from build123d import *

# Parameters (mm, degrees)
POCKET_DEPTH       = 34.402163
POCKET_DEPTH_BACK  = 40.002163
POLARPATTERN_COUNT = 6


with BuildPart() as part:
    # Sketch → Revolution (revolve)
    with BuildSketch(Plane.XZ):
        Polygon((-3.6, 4.6), (-3.6, 3.5), (-3.38, 3), (-3.6, 2.5), (-3.6, 1), (-3.405, 0.5), (-3.905, 0), (-4.4, 0), (-5.4, 0), (-5.75, 0.35), (-5.75, 1), (-4.675, 1), (-4.675, 2.3), (-4.4, 2.575), (-4.4, 4.85), (-3.65, 5.6), (-3.15, 5.6), (-2.975, 5.1), (-3.15, 4.6), align=None)
    revolve(axis=Axis((0, 0, 0), (0, 0, 1)))

    # Sketch001 → Pocket (cut, two sides)
    with BuildSketch(Plane.XY) as pocket_sk:
        with BuildLine():
            Line((0, 0), (-0.776457, 2.897777))
            ThreePointArc((-0.587735, 3.196415), (-0.747472, 3.08841), (-0.776457, 2.897777))
            ThreePointArc((0.587735, 3.196415), (0, 3.25), (-0.587735, 3.196415))
            ThreePointArc((0.776457, 2.897777), (0.747472, 3.08841), (0.587735, 3.196415))
            Line((0.776457, 2.897777), (0, 0))
        make_face()
    pocket = extrude(amount=-POCKET_DEPTH, mode=Mode.SUBTRACT) + extrude(pocket_sk.sketch, amount=POCKET_DEPTH_BACK, mode=Mode.SUBTRACT)

    # PolarPattern: Pocket ×6 about axis
    polarpattern_axis = Axis((0, 0, 0), (0, 0, 1))
    for i in range(1, POLARPATTERN_COUNT):
        add(pocket.rotate(polarpattern_axis, i * 360 / POLARPATTERN_COUNT), mode=Mode.SUBTRACT)


solid = part.part
Input: part model. Units: mm. Frame: model coordinates. A direction names the side the tool comes from. Coordinates: 2 decimals unless noted, no trailing zeros. Loops run counter-clockwise (first coordinate to the right, second up) from the corner with the lowest first, then second, coordinate; pieces in that order, holes last.
Q1. Cut plane B-B (z = 4.45). Output: boundary loops of the cut face in (x, y), then the cut area to 3 significant figures.
Q2. Contact query for flat-ended pins moving along their axis: pin 1 (2 mm diameter, centred on x = 1, y = -1.5, fed in from -Z); pin 2 (1 mm diameter, centred on y = -4.5, z = 3, fed in from +X); pin 3 (1.5 mm diameter, centred on x = 0.5, z = 5, fed in from -Y); pin 4 (1 mm diameter, centred on x = 1.5, y = -4.5, fed in from +Z). Output: stop coordinate, or through.
Q3. Draft query along Z for faces 1 (the face through (1.013, 4.564, 1.659)), 2 (the face through (-3.434, -1.081, 1.74)), 3 (the face through (-3.434, -1.081, 4.042)), 4 (the face through (-1.542, -2.647, 4.846)). Return one class per face: +Z half, -Z half, draft (parallel to the pull), parting line (faces both ways), or undercut.
Q4. Set-up query: faces 5 (the face through (-4.197, -1.322, 3.728)), 6 (the face through (0.01, 3.25, 5.09)), 7 (the face through (1.542, 2.647, 4.846)). Return all of +Z, -Z, +X, -X, +Y, -Y with unobstructed straight access to the full face (end or side cutting, diameter ignored); none if empty.
Q5. Cut plane C-C (z = 3.15). Output: boundary loops of the cut face in (x, y).
Q6. Material intervals for line 1 (X direction, y = 0, z = 3.95); line 2 (X direction, y = 0, z = 2.05) (3 decimals); line 3 (Z direction, x = 1.25, y = -3.25), sorted ascending.
Working result:
1. outline: circle Ø8.8 at (0, 0); hole circle Ø7.2 at (0, 0)
1. area: 20.1 mm2
2. pin 1: passes through
2. pin 2: stops at x = 1.83
2. pin 3: stops at y = -4.4
2. pin 4: stops at z = 5.01
3. face 1: draft
3. face 2: undercut
3. face 3: undercut
3. face 4: -Z half
4. face 5: +Z
4. face 6: +Z, -Z
4. face 7: -Z
5. outline: circle Ø8.8 at (0, 0); hole circle Ø6.89 at (0, 0)
6. line 1: x = -4.4 to -3.6, 3.6 to 4.4
6. line 2: x = -4.675 to -3.6, 3.6 to 4.675
6. line 3: z = 0.42 to 0.7, 2.77 to 3.23, 4.6 to 5.6
